The drawing under review shows one solid part. Ordinate dimensions are in mm from its lowest x, y, z. A direction names the side the tool comes from. Round coordinates to 2 decimals unless told otherwise and drop trailing zeros. Write each loop counter-clockwise with the first axis right and the second up, starting at its lowest first coordinate (ties: lowest second). Pieces come first, ordered by that corner, then holes. Notation, with made-up numbers: (44.25, 27.25) -> (80.25, 27.25) arc R27 ccw to (80.25, 66.25) -> close; hole circle Ø7 at (55, 4). An arc over 180 degrees is marked (long way). Answer in a Markdown table with one row per item.
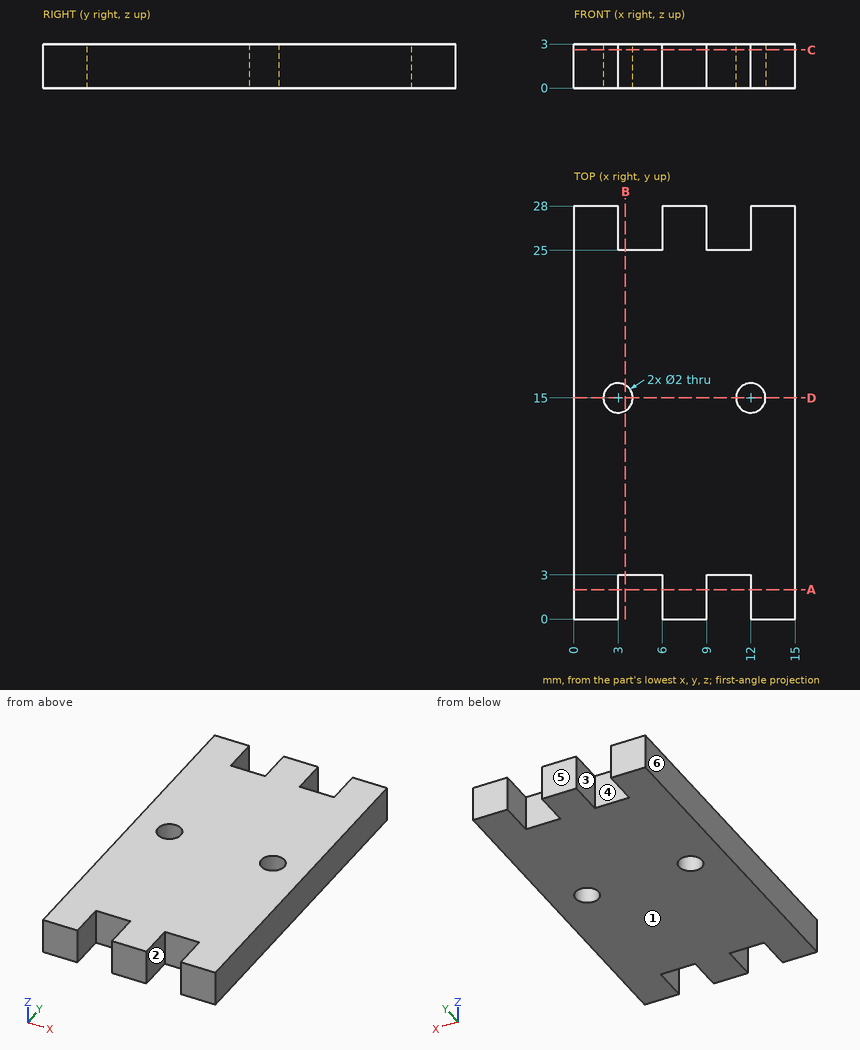
1) Consider section C-C on z = 2.6. State the section outline as (x, y) points.
Solved:
| item | result |
|---|---|
| outline | (0, 0) -> (3, 0) -> (3, 3) -> (6, 3) -> (6, 0) -> (9, 0) -> (9, 3) -> (12, 3) -> (12, 0) -> (15, 0) -> (15, 28) -> (12, 28) -> (12, 25) -> (9, 25) -> (9, 28) -> (6, 28) -> (6, 25) -> (3, 25) -> (3, 28) -> (0, 28) -> close; hole circle Ø2 at (3, 15); hole circle Ø2 at (12, 15) |
2) Consider section D-D on y = 15. State the section outline as (x, z) points, then the cut area to 3 significant figures.
Solved:
| item | result |
|---|---|
| outline | (0, 0) -> (2, 0) -> (2, 3) -> (0, 3) -> close; (4, 0) -> (11, 0) -> (11, 3) -> (4, 3) -> close; (13, 0) -> (15, 0) -> (15, 3) -> (13, 3) -> close |
| area | 33.0 mm² |
3) Mouldability with a two-part tool opening along X and no side actions: class the marked faces 4, 5 and 6 as pulls with the +X half, pulls with the -X half, needs draft (parallel to the pull), parting line crosses it, or undercut.
Solved:
| item | result |
|---|---|
| face 4 | undercut |
| face 5 | needs draft |
| face 6 | pulls with the -X half |
4) For line 1 (X direction, y = 2, z = 2.75); line 2 (X direction, y = 14.75, z = 2.85); line 3 (Y direction, x = 9.5, z = 0.95), list the stretches that pass through material, from the lowest coordinate up. Write a range as [from, to].
Solved:
| item | result |
|---|---|
| line 1 | [0, 3], [6, 9], [12, 15] |
| line 2 | [0, 2.03], [3.97, 11.03], [12.97, 15] |
| line 3 | [3, 25] |
5) For the marked faces 1, 2 and 3, list the 3-axis set-ups (+Z, -Z, +X, -X, +Y, -Y) from which the entire face can be reached by the end or side of a thin tool; tool diameter is ignored.
Solved:
| item | result |
|---|---|
| face 1 | -Z, +X, -X, +Y, -Y |
| face 2 | +Z, -Z, -Y |
| face 3 | +Z, -Z, +Y |
6) Consider section A-A on y = 2. State the section outline as (x, z) points.
Solved:
| item | result |
|---|---|
| outline | (0, 0) -> (3, 0) -> (3, 3) -> (0, 3) -> close; (6, 0) -> (9, 0) -> (9, 3) -> (6, 3) -> close; (12, 0) -> (15, 0) -> (15, 3) -> (12, 3) -> close |
7) Clearance check with flat-ended pins moving along their axes: pin 1 Ø1.5 at (x, z) = (4.5, 1.5) entering from +Y; pin 2 Ø0.9 at (x, z) = (5, 2) entering from -Y. State where each tip first meets the part, or that it passes through.
Solved:
| item | result |
|---|---|
| pin 1 | y = 25 |
| pin 2 | y = 3 |
8) Consider section B-B on x = 3.5. State the section outline as (y, z) points.
Solved:
| item | result |
|---|---|
| outline | (3, 0) -> (14.13, 0) -> (14.13, 3) -> (3, 3) -> close; (15.87, 0) -> (25, 0) -> (25, 3) -> (15.87, 3) -> close |
